from build123d import *

# Parameters (mm, degrees)
SKETCH1_R               = 15
SKETCH1_R_2             = 1.55
BOSS_EXTRUDE1_DEPTH     = 2.5
BOSS_EXTRUDE2_START     = 2.5
SKETCH3_R               = 7.5
BOSS_EXTRUDE2_DEPTH     = 9.3
CUT_EXTRUDE1_DEPTH      = 25.274266209
CUT_EXTRUDE1_DEPTH_BACK = 25.274266209
SKETCH4_R               = 2.5
SKETCH5_R               = 5
CUT_EXTRUDE2_DEPTH      = 5.5
CUT_EXTRUDE3_DEPTH      = 25.274266209
CUT_EXTRUDE3_DEPTH_BACK = 25.274266209
SKETCH6_R               = 1.85


with BuildPart() as part:
    # Sketch1 → Boss-Extrude1 (new body)
    with BuildSketch(Plane.XY):
        Circle(SKETCH1_R)
        with Locations((0, 12.5)):
            Circle(SKETCH1_R_2, mode=Mode.SUBTRACT)
        with Locations((12.5, 0)):
            Circle(SKETCH1_R_2, mode=Mode.SUBTRACT)
        with Locations((0, -12.5)):
            Circle(SKETCH1_R_2, mode=Mode.SUBTRACT)
        with Locations((-12.5, 0)):
            Circle(SKETCH1_R_2, mode=Mode.SUBTRACT)
    extrude(amount=BOSS_EXTRUDE1_DEPTH)

    # Sketch3 → Boss-Extrude2 (add)
    with BuildSketch(Plane.XY.offset(BOSS_EXTRUDE2_START)):
        Circle(SKETCH3_R)
    extrude(amount=BOSS_EXTRUDE2_DEPTH)

    # Sketch4 → Cut-Extrude1 (cut, two sides: drawn at the far end of the back side and taken through both)
    with BuildSketch(Plane.XY.offset(11.8).offset(-CUT_EXTRUDE1_DEPTH_BACK)):
        Circle(SKETCH4_R)
    extrude(amount=CUT_EXTRUDE1_DEPTH + CUT_EXTRUDE1_DEPTH_BACK, mode=Mode.SUBTRACT)

    # Sketch5 → Cut-Extrude2 (cut)
    with BuildSketch(Plane.XY.offset(11.8)):
        Circle(SKETCH5_R)
    extrude(amount=-CUT_EXTRUDE2_DEPTH, mode=Mode.SUBTRACT)

    # Sketch6 → Cut-Extrude3 (cut, two sides: drawn at the far end of the back side and taken through both)
    with BuildSketch(Plane(origin=(0, 0, 0), x_dir=(1, 0, 0), z_dir=(0, 1, 0)).offset(-CUT_EXTRUDE3_DEPTH_BACK)):
        with Locations(Location((0, -9.3, 0), (0, 0, 270))):
            Circle(SKETCH6_R)
    extrude(amount=CUT_EXTRUDE3_DEPTH + CUT_EXTRUDE3_DEPTH_BACK, mode=Mode.SUBTRACT)


solid = part.part
Read the model definition and answer for the solid it produces. Units are mm, in the model's axes. A direction names the side the tool comes from. Round coordinates to 2 decimals unless told otherwise and drop trailing zeros. Write each loop counter-clockwise with the first axis right and the second up, starting at its lowest first coordinate (ties: lowest second). Pieces come first, ordered by that corner, then holes. Notation, with made-up numbers: (15.5, 83) - (22.5, 83) arc R35 cw to (22.5, 120) - close; hole circle Ø9 at (62.5, 23). An arc over 180 degrees is marked (long way). Use a Markdown table: item, result.
(1) The part is cut by section B-B (x = 0). State how many separate pieces and enclosed holes the cut face has, then the cut area to 3 significant figures.
Reported:
| item | result |
|---|---|
| separate pieces | 6 |
| enclosed holes | 0 |
| area | 94.0 mm2 |
(2) The part is cut by section D-D (y = 13). Write down the section's boundary in (x, z), then the cut area to 3 significant figures.
Reported:
| item | result |
|---|---|
| outline | (-7.48, 0) - (-1.47, 0) - (-1.47, 2.5) - (-7.48, 2.5) - close; (1.47, 0) - (7.48, 0) - (7.48, 2.5) - (1.47, 2.5) - close |
| area | 30.1 mm2 |
(3) Each of these flat-tipped pins is pushed along its axis until it touches: pin 1 Ø9 at (x, y) = (0, 0) entering from +Z; pin 2 Ø3 at (y, z) = (1.5, 8.5) entering from -X; pin 3 Ø5 at (x, y) = (12.5, 0) entering from +Z. Where does it stop, or does it pass through?
Reported:
| item | result |
|---|---|
| pin 1 | z = 6.3 |
| pin 2 | x = -7.5 |
| pin 3 | z = 2.5 |
(4) Straight lines are drawn through the part: line 1 along Z through (x, y) = (0, -6.2); line 2 along X through (y, z) = (1, 1); line 3 along Z through (x, y) = (12.25, 6). For each, find the intervals that lie inside material, in ascending order. Write a range as [from, to].
Reported:
| item | result |
|---|---|
| line 1 | [0, 7.45], [11.15, 11.8] |
| line 2 | [-14.97, -13.68], [-11.32, -2.29], [2.29, 11.32], [13.68, 14.97] |
| line 3 | [0, 2.5] |
(5) The part is cut by section C-C (x = 12.5). Write down the section's boundary in (y, z), then the cut area to 3 significant figures.
Reported:
| item | result |
|---|---|
| outline | (-8.29, 0) - (-1.55, 0) - (-1.55, 2.5) - (-8.29, 2.5) - close; (1.55, 0) - (8.29, 0) - (8.29, 2.5) - (1.55, 2.5) - close |
| area | 33.7 mm2 |
(6) Which of the six approach directions +Z, -Z, +X, -X, +Y, -Y give full straight-line access (tool end or side, diameter ignored) to faces 4 (the flat face through (2, -2, 6.3)), 5 (the cylindrical face through (-14.985, 0.66, 1.232))?
Reported:
| item | result |
|---|---|
| face 4 | +Z |
| face 5 | +Z, -Z |
(7) The mould has two halves that part along X. Classify faces 1 (the flat face through (-4, 7, 2.5)), 2 (the cylindrical face through (3.461, -6.654, 7.085)), 3 (the cylindrical face through (1.56, 6.055, 10.295)): released by +X, released by -X, zero draft, split by the parting line, or undercut.
Reported:
| item | result |
|---|---|
| face 1 | zero draft |
| face 2 | split by the parting line |
| face 3 | undercut |
(8) The part is cut by section A-A (y = 0). Write down the section's boundary in (x, z).
Reported:
| item | result |
|---|---|
| outline | (-15, 0) - (-14.05, 0) - (-14.05, 2.5) - (-15, 2.5) - close; (-10.95, 0) - (-2.5, 0) - (-2.5, 6.3) - (-5, 6.3) - (-5, 11.8) - (-7.5, 11.8) - (-7.5, 2.5) - (-10.95, 2.5) - close; (2.5, 0) - (10.95, 0) - (10.95, 2.5) - (7.5, 2.5) - (7.5, 11.8) - (5, 11.8) - (5, 6.3) - (2.5, 6.3) - close; (14.05, 0) - (15, 0) - (15, 2.5) - (14.05, 2.5) - close |
